Source: CAD feature listing. Evaluate the final solid. Frame: model axes, mm. Coordinates: 2 decimals unless noted, no trailing zeros. Write each loop counter-clockwise with the first axis right and the second up, starting at its lowest first coordinate (ties: lowest second). Pieces come first, ordered by that corner, then holes. Notation, with made-up numbers: (6, -32.75) - (44, -32.75) arc R25 ccw to (44, -6.75) - close; hole circle Ø8 at (4, 30.25). An arc over 180 degrees is marked (long way). One line per item, written item: value.
Autodesk Inventor part; units mm, degrees
ref_plane "YZ Plane" through (0, 0, 0) normal (1, 0, 0) x (0, 1, 0)
ref_plane "XZ Plane" through (0, 0, 0) normal (0, 1, 0) x (-1, 0, 0)
ref_plane "XY Plane" through (0, 0, 0) normal (0, 0, 1) x (1, 0, 0)
sketch "Sketch1" plane through (0, 0, 0) normal (0, 1, 0) x (-1, 0, 0)
  line L0 (-113.5, -45) -> (113.5, -45)
  line L1 (115, -44) -> (115, 44)
  line L2 (113.5, 45) -> (-113.5, 45)
  line L3 (-115, 44) -> (-115, -44)
  circle A0 centre (0, 0) radius 5
  line L4 (-113.5, -45) -> (-115, -44)
  line L5 (-115, 44) -> (-113.5, 45)
  line L6 (115, 44) -> (113.5, 45)
  line L7 (115, -44) -> (113.5, -45)
  circle A1 centre (-94, -30) radius 5
  circle A2 centre (-94, 30) radius 5
  line L8 (0, 45) -> (0, -45) construction
  circle A3 centre (94, -30) radius 5
  circle A4 centre (94, 30) radius 5
  point P0 (-115, -45)
  point P1 (115, 45)
  point P2 (115, -45)
  point P3 (-115, 45)
  point P4 (115, 0)
  dimension "d0" = 230
  dimension "d1" = 90
  dimension "d2" = 115
  dimension "d3" = 45
  dimension "d6" = 10
  dimension "d7" = 1.5
  dimension "d8" = 1
  dimension "d9" = 1
  dimension "d10" = 1.5
  dimension "d11" = 1
  dimension "d12" = 1.5
  dimension "d13" = 1
  dimension "d14" = 1.5
  dimension "d15" = 10
  dimension "d16" = 10
  dimension "d17" = 30
  dimension "d18" = 30
  dimension "d19" = 94
  dimension "d20" = 94
extrude "Extrusion1" add sketch "Sketch1" along normal blind 6
equation "\"plate_thick\" = 6"
equation "\"plates_spacing\" = 116"
properties part number "rig_connector"
1) Draft query along Z for faces 1 (the cylindrical face through (89.381, 2.958, 31.915)), 2 (the flat face through (2, 3, -45)), 3 (the flat face through (115, 3, 1)). Return one class per face: released by +Z, released by -Z, zero draft, split by the parting line, or undercut.
Values found:
face 1: undercut
face 2: released by -Z
face 3: zero draft
2) Section query C-C on y = 4.9. Output: boundary loops of the cut face in (x, z), then the cut area to 3 significant figures.
Values found:
outline: (-115, -44) - (-113.5, -45) - (113.5, -45) - (115, -44) - (115, 44) - (113.5, 45) - (-113.5, 45) - (-115, 44) - close; hole circle Ø10 at (-94, -30); hole circle Ø10 at (-94, 30); hole circle Ø10 at (0, 0); hole circle Ø10 at (94, -30); hole circle Ø10 at (94, 30)
area: 20,300 mm2
3) Section query A-A on z = 0. Output: boundary loops of the cut face in (x, y), then the cut area to 3 significant figures.
Values found:
outline: (-115, 0) - (-5, 0) - (-5, 6) - (-115, 6) - close; (5, 0) - (115, 0) - (115, 6) - (5, 6) - close
area: 1,320 mm2
4) Contact query for a flat-ended pin moving along its axis: P1, Ø9, axis at x = 0, z = 0, coming from the +Y side. Output: stop coordinate, or through.
Values found:
P1: through
5) Section query D-D on x = 0. Output: boundary loops of the cut face in (y, z), then the cut area to 3 significant figures.
Values found:
outline: (0, -45) - (6, -45) - (6, -5) - (0, -5) - close; (0, 5) - (6, 5) - (6, 45) - (0, 45) - close
area: 480 mm2
6) Section query B-B on x = 94. Output: boundary loops of the cut face in (y, z), then the cut area to 3 significant figures.
Values found:
outline: (0, -45) - (6, -45) - (6, -35) - (0, -35) - close; (0, -25) - (6, -25) - (6, 25) - (0, 25) - close; (0, 35) - (6, 35) - (6, 45) - (0, 45) - close
area: 420 mm2
7) Material intervals for line 1 (Z direction, x = 94, y = 3.15); line 2 (Z direction, x = 95, y = 4.55); line 3 (X direction, y = 2.05, z = -1.5), sorted ascending.
Values found:
line 1: -45 to -35, -25 to 25, 35 to 45
line 2: -45 to -34.9, -25.1 to 25.1, 34.9 to 45
line 3: -115 to -4.77, 4.77 to 115
